The listing builds one solid part. Answer for the finished solid, in the listing's coordinates (mm). A direction names the side the tool comes from. Round coordinates to 2 decimals unless told otherwise and drop trailing zeros. Write each loop counter-clockwise with the first axis right and the second up, starting at its lowest first coordinate (ties: lowest second). Pieces come first, ordered by that corner, then holes.
Item 1: Find section B-B on z = 23.5. Give the vertices of the cut face in (x, y), then the cut area to 3 significant figures.
Item 2: Find section D-D on z = 43. Give the vertices of the cut face in (x, y), then the cut area to 3 significant figures.
Item 3: Find section C-C on y = 0. Give the vertices of the cut face in (x, z), then the cut area to 3 significant figures.
Item 4: For a pull along Y with two mould halves and no side action, classify faces 1 (the face through (15, 0, 26)), 2 (the face through (-14.57, -14.55, 26.87)), 3 (the face through (-5, 0, 43)) as +Y half, -Y half, draft (parallel to the pull), parting line (faces both ways), or undercut.
Item 5: Find section A-A on x = -8. Give the vertices of the cut face in (y, z).
Item 6: Find the intervals of material crossed by probe 1 along Z at (x, y) = (8, 12.5); probe 2 along Z at (x, y) = (7.75, -3.25); probe 3 along X at (y, z) = (10, 7), in increasing order.
Item 7: A tool of negligible diameter and unlimited length cuts with its end or side. For faces 4 (the face through (4.86, 0.96, 40.69)), 5 (the face through (-4.095, -3.339, 7.867)), 6 (the face through (-5.87, 11.45, 7.28)), from which of +Z, -Z, +X, -X, +Y, -Y can it reach the whole face along a straight path? Write none if from no direction.
Item 8: Each of these flat-tipped pins is pushed along its axis until it touches: pin 1 (6.5 mm diameter, centred on x = 8, z = 7, fed in from -Y); pin 2 (4 mm diameter, centred on y = 0, z = 43, fed in from +X). Where does it stop, or does it pass through?
Solid Edge part; units mm, degrees
sketch "Sketch1" plane through (0, 0, 0) normal (0, 0, 1) x (1, 0, 0)
  line L0 (-15, -15) -> (15, -15)
  line L1 (15, -15) -> (15, 15)
  line L2 (15, 15) -> (-15, 15)
  line L3 (-15, 15) -> (-15, -15)
extrude "Protrusion1" add sketch "Sketch1" along normal blind 53
hole "Hole_1" at (-8, -15, 23.5) direction (0, 1, 0) diameter 4.3 end up to next counterbore diameter 8 counterbore depth 23
hole "Hole1" at (8, -15, 23.5) direction (0, 1, 0) diameter 4.3 end up to next counterbore diameter 8 counterbore depth 23
hole "Hole2" at (8, -15, 7) direction (0, 1, 0) diameter 4.3 end up to next counterbore diameter 8 counterbore depth 23
hole "Hole3" at (-8, -15, 7) direction (0, 1, 0) diameter 4.3 end up to next counterbore diameter 8 counterbore depth 23
hole "Hole_5" at (15, 0, 43) direction (-1, 0, 0) diameter 5 depth 20
fillet "Round_1" radius 1.5 4 edges at (-15, -15, 26.5) (15, -15, 26.5) (-15, 15, 26.5) (15, 15, 26.5)
properties material "POM"
Check values:
1. outline: (-15, -13.5) arc R1.5 ccw to (-13.5, -15) - (-12, -15) - (-12, 8) - (-10.15, 8) - (-10.15, 15) - (-13.5, 15) arc R1.5 ccw to (-15, 13.5) - close; (-5.85, 8) - (-4, 8) - (-4, -15) - (4, -15) - (4, 8) - (5.85, 8) - (5.85, 15) - (-5.85, 15) - close; (10.15, 8) - (12, 8) - (12, -15) - (13.5, -15) arc R1.5 ccw to (15, -13.5) - (15, 13.5) arc R1.5 ccw to (13.5, 15) - (10.15, 15) - close
1. area: 470 mm2
2. outline: (-15, -13.5) arc R1.5 ccw to (-13.5, -15) - (13.5, -15) arc R1.5 ccw to (15, -13.5) - (15, -2.5) - (-5, -2.5) - (-5, 2.5) - (15, 2.5) - (15, 13.5) arc R1.5 ccw to (13.5, 15) - (-13.5, 15) arc R1.5 ccw to (-15, 13.5) - close
2. area: 798 mm2
3. outline: (-15, 0) - (15, 0) - (15, 40.5) - (-5, 40.5) - (-5, 45.5) - (15, 45.5) - (15, 53) - (-15, 53) - close; hole circle Ø8 at (-8, 7); hole circle Ø8 at (-8, 23.5); hole circle Ø8 at (8, 7); hole circle Ø8 at (8, 23.5)
3. area: 1,290 mm2
4. face 1: draft
4. face 2: -Y half
4. face 3: undercut
5. outline: (-15, 0) - (15, 0) - (15, 4.85) - (8, 4.85) - (8, 3) - (-15, 3) - close; (-15, 11) - (8, 11) - (8, 9.15) - (15, 9.15) - (15, 21.35) - (8, 21.35) - (8, 19.5) - (-15, 19.5) - close; (-15, 27.5) - (8, 27.5) - (8, 25.65) - (15, 25.65) - (15, 53) - (-15, 53) - close
6. probe 1: z = 0 to 4.85, 9.15 to 21.35, 25.65 to 53
6. probe 2: z = 0 to 3.01, 10.99 to 19.51, 27.49 to 53
6. probe 3: x = -15 to -10.15, -5.85 to 5.85, 10.15 to 15
7. face 4: +X
7. face 5: -Y
7. face 6: +Y, -Y
8. pin 1: stops at y = 8
8. pin 2: stops at x = -5
